Build history of the part. All positions in model axes, mm. A direction names the side the tool comes from. Coordinates: 2 decimals unless noted, no trailing zeros. Loops run counter-clockwise (first coordinate to the right, second up) from the corner with the lowest first, then second, coordinate; pieces in that order, holes last.
Item 1: Drill centre lines: line 1 along Z through (x, y) = (-53.34, -3.75) (3 decimals); line 2 along Z through (x, y) = (-45.72, -4.5) (3 decimals); line 3 along X through (y, z) = (-5.5, -33.5). Where is each one in solid material? Low to high.
Item 2: Cut at A-A (y = -4.5). Count the separate pieces of the cut face and the enclosed holes in it, and give its area (3 significant figures).
Item 3: Flat gauge pins, fed straight in: pin 1 (0.5 mm diameter, centred on y = -2, z = -53.5, fed in from +X); pin 2 (1.5 mm diameter, centred on y = -1, z = 51.5, fed in from +X); pin 3 (3 mm diameter, centred on x = 18, y = -3.5, fed in from +Z) (3 decimals). Where does each tip first touch, or does it go through?
Item 4: Cut at B-B (z = 45.5). List the corners of the cut face in (x, y), and give its area (3 significant figures).
Item 5: Cut at C-C (x = -17). List the corners of the cut face in (y, z) (3 decimals).
Item 6: Mould opens along X. For faces 6 (the face through (-1, -3, 70.485)), 7 (the face through (62, -3, -49.708)), 8 (the face through (63.5, -3, -45)) say: released by +X, released by -X, zero draft, split by the parting line, or undercut.
Item 7: 3-axis set-ups, long thin cutter, end or side, ignore diameter. For faces 1 (the face through (63.5, -3, -63)), 2 (the face through (-62, -3, 52.908)), 3 (the face through (63.5, -3, 45)), 4 (the face through (-56.2, -3.13, -37.19)), 5 (the face through (-63.5, -3, -45)): which of +Z, -Z, +X, -X, +Y, -Y reach the whole face in a straight line?
from build123d import *

# Parameters (mm, degrees)
SKETCH1_R           = 0.4
BOSS_EXTRUDE1_DEPTH = 6.35
SKETCH5_R           = 1.25
CUT_EXTRUDE3_DEPTH  = 6.35
SKETCH4_W           = 3.2
SKETCH4_H           = 6.35
CUT_EXTRUDE4_DEPTH  = 11.43
SKETCH2_W           = 3.2
SKETCH2_H           = 6.35
CUT_EXTRUDE5_DEPTH  = 11.43
FILLET1_R           = 1.27
SKETCH6_W           = 3.81
SKETCH6_H           = 6
CUT_EXTRUDE6_DEPTH  = 6.35
FILLET2_R           = 0.762


with BuildPart() as part:
    # Sketch1 → Boss-Extrude1 (new body)
    with BuildSketch(Plane(origin=(0, 0, 0), x_dir=(1, 0, 0), z_dir=(0, 1, 0))):
        with BuildLine():
            Line((-60.325, -75.565), (-39.37, -75.565))
            ThreePointArc((-39.37, -75.565), (-38.471974388, -75.193025612), (-38.1, -74.295))
            Line((-38.1, -74.295), (-38.1, -71.755))
            ThreePointArc((-38.1, -71.755), (-37.728025612, -70.856974388), (-36.83, -70.485))
            Line((-36.83, -70.485), (36.83, -70.485))
            ThreePointArc((36.83, -70.485), (37.728025612, -70.856974388), (38.1, -71.755))
            Line((38.1, -71.755), (38.1, -74.295))
            ThreePointArc((38.1, -74.295), (38.471974388, -75.193025612), (39.37, -75.565))
            Line((39.37, -75.565), (60.325, -75.565))
            ThreePointArc((60.325, -75.565), (62.57006403, -74.63506403), (63.5, -72.39))
            Line((63.5, -72.39), (63.5, -40.64))
            ThreePointArc((63.5, -40.64), (64.243948776, -38.843948776), (66.04, -38.1))
            Line((66.04, -38.1), (67.31, -38.1))
            ThreePointArc((67.31, -38.1), (69.106051224, -37.356051224), (69.85, -35.56))
            Line((69.85, -35.56), (69.85, 35.56))
            ThreePointArc((69.85, 35.56), (69.106051224, 37.356051224), (67.31, 38.1))
            Line((67.31, 38.1), (66.04, 38.1))
            ThreePointArc((66.04, 38.1), (64.243948776, 38.843948776), (63.5, 40.64))
            Line((63.5, 40.64), (63.5, 72.39))
            ThreePointArc((63.5, 72.39), (62.57006403, 74.63506403), (60.325, 75.565))
            Line((60.325, 75.565), (39.37, 75.565))
            ThreePointArc((39.37, 75.565), (38.471974388, 75.193025612), (38.1, 74.295))
            Line((38.1, 74.295), (38.1, 71.755))
            ThreePointArc((38.1, 71.755), (37.728025612, 70.856974388), (36.83, 70.485))
            Line((36.83, 70.485), (-36.83, 70.485))
            ThreePointArc((-36.83, 70.485), (-37.728025612, 70.856974388), (-38.1, 71.755))
            Line((-38.1, 71.755), (-38.1, 74.295))
            ThreePointArc((-38.1, 74.295), (-38.471974388, 75.193025612), (-39.37, 75.565))
            Line((-39.37, 75.565), (-60.325, 75.565))
            ThreePointArc((-60.325, 75.565), (-62.57006403, 74.63506403), (-63.5, 72.39))
            Line((-63.5, 72.39), (-63.5, 40.64))
            ThreePointArc((-63.5, 40.64), (-64.243948776, 38.843948776), (-66.04, 38.1))
            Line((-66.04, 38.1), (-67.31, 38.1))
            ThreePointArc((-67.31, 38.1), (-69.106051224, 37.356051224), (-69.85, 35.56))
            Line((-69.85, 35.56), (-69.85, -35.56))
            ThreePointArc((-69.85, -35.56), (-69.106051224, -37.356051224), (-67.31, -38.1))
            Line((-67.31, -38.1), (-66.04, -38.1))
            ThreePointArc((-66.04, -38.1), (-64.243948776, -38.843948776), (-63.5, -40.64))
            Line((-63.5, -40.64), (-63.5, -72.39))
            ThreePointArc((-63.5, -72.39), (-62.57006403, -74.63506403), (-60.325, -75.565))
        make_face()
        with Locations(Location((-45.72, 70.485, 0), (0, 0, 270))):
            Circle(SKETCH1_R, mode=Mode.SUBTRACT)
        with Locations(Location((-43.18, 70.485, 0), (0, 0, 270))):
            Circle(SKETCH1_R, mode=Mode.SUBTRACT)
        with Locations(Location((-55.88, 70.485, 0), (0, 0, 270))):
            Circle(SKETCH1_R, mode=Mode.SUBTRACT)
        with Locations(Location((-53.34, 70.485, 0), (0, 0, 270))):
            Circle(SKETCH1_R, mode=Mode.SUBTRACT)
        with BuildLine():
            Line((-53.975, -38.1), (-41.275, -38.1))
            ThreePointArc((-41.275, -38.1), (-39.02993597, -37.17006403), (-38.1, -34.925))
            Line((-38.1, -34.925), (-38.1, 34.925))
            ThreePointArc((-38.1, 34.925), (-39.02993597, 37.17006403), (-41.275, 38.1))
            Line((-41.275, 38.1), (-53.975, 38.1))
            ThreePointArc((-53.975, 38.1), (-56.22006403, 37.17006403), (-57.15, 34.925))
            Line((-57.15, 34.925), (-57.15, -34.925))
            ThreePointArc((-57.15, -34.925), (-56.22006403, -37.17006403), (-53.975, -38.1))
        make_face(mode=Mode.SUBTRACT)
    extrude(amount=-BOSS_EXTRUDE1_DEPTH)

    # Sketch5 → Cut-Extrude3 (cut)
    with BuildSketch(Plane(origin=(0, 0, 0), x_dir=(1, 0, 0), z_dir=(0, 1, 0))):
        with Locations(Location((-11.8, -4.235, 0), (0, 0, 270))):
            Circle(SKETCH5_R)
        with Locations(Location((-11.8, 53.765, 0), (0, 0, 270))):
            Circle(SKETCH5_R)
        with Locations(Location((37.2, -4.235, 0), (0, 0, 270))):
            Circle(SKETCH5_R)
        with Locations(Location((37.2, 53.765, 0), (0, 0, 270))):
            Circle(SKETCH5_R)
    extrude(amount=-CUT_EXTRUDE3_DEPTH, mode=Mode.SUBTRACT)

    # Sketch4 → Cut-Extrude4 (cut)
    with BuildSketch(Plane.ZY.offset(63.5)):
        with Locations((51.308, -3.175)):
            Rectangle(SKETCH4_W, SKETCH4_H)
        with Locations((-51.308, -3.175)):
            Rectangle(SKETCH4_W, SKETCH4_H)
    extrude(amount=-CUT_EXTRUDE4_DEPTH, mode=Mode.SUBTRACT)

    # Sketch2 → Cut-Extrude5 (cut)
    with BuildSketch(Plane(origin=(63.5, 0, 0), x_dir=(0, 0, -1), z_dir=(1, 0, 0))):
        with Locations((51.308, -3.175)):
            Rectangle(SKETCH2_W, SKETCH2_H)
        with Locations((-51.308, -3.175)):
            Rectangle(SKETCH2_W, SKETCH2_H)
    extrude(amount=-CUT_EXTRUDE5_DEPTH, mode=Mode.SUBTRACT)

    # Fillet1
    fillet1_edges = [part.edges().sort_by_distance(p)[0] for p in [
        (-52.07, -3.175, 49.708),
        (-52.07, -3.175, 52.908),
        (-52.07, -3.175, -52.908),
        (-52.07, -3.175, -49.708),
        (52.07, -3.175, -49.708),
        (52.07, -3.175, -52.908),
        (52.07, -3.175, 52.908),
        (52.07, -3.175, 49.708),
    ]]
    fillet(fillet1_edges, radius=FILLET1_R)

    # Sketch6 → Cut-Extrude6 (cut)
    with BuildSketch(Plane(origin=(0, 0, 0), x_dir=(1, 0, 0), z_dir=(0, 1, 0))):
        with Locations((57.785, -51.308)):
            Rectangle(SKETCH6_W, SKETCH6_H)
        with Locations((-57.785, -51.308)):
            Rectangle(SKETCH6_W, SKETCH6_H)
        with Locations((-57.785, 51.308)):
            Rectangle(SKETCH6_W, SKETCH6_H)
        with Locations((57.785, 51.308)):
            Rectangle(SKETCH6_W, SKETCH6_H)
    extrude(amount=-CUT_EXTRUDE6_DEPTH, mode=Mode.SUBTRACT)

    # Fillet2
    fillet2_edges = [part.edges().sort_by_distance(p)[0] for p in [
        (55.88, -3.175, -48.308),
        (59.69, -3.175, -54.308),
        (59.69, -3.175, -48.308),
        (55.88, -3.175, -54.308),
        (-55.88, -3.175, -54.308),
        (-59.69, -3.175, -48.308),
        (-59.69, -3.175, -54.308),
        (-55.88, -3.175, -48.308),
        (-55.88, -3.175, 48.308),
        (-59.69, -3.175, 48.308),
        (-55.88, -3.175, 54.308),
        (-59.69, -3.175, 54.308),
        (55.88, -3.175, 54.308),
        (59.69, -3.175, 48.308),
        (55.88, -3.175, 48.308),
        (59.69, -3.175, 54.308),
    ]]
    fillet(fillet2_edges, radius=FILLET2_R)


solid = part.part
Filled sheet:
1. line 1: z = -75.565 to -70.885, -70.085 to -52.908, -49.708 to -38.1, 38.1 to 49.708, 52.908 to 75.565
1. line 2: z = -75.565 to -70.885, -70.085 to -38.1, 38.1 to 75.565
1. line 3: x = -69.85 to -57.15, -38.1 to 69.85
2. separate pieces: 1
2. enclosed holes: 9
2. area: 17,700 mm2
3. pin 1: stops at x = 63.5
3. pin 2: stops at x = 52.23
3. pin 3: stops at z = 70.485
4. outline: (-63.5, -6.35) - (63.5, -6.35) - (63.5, 0) - (-63.5, 0) - close
4. area: 806 mm2
5. outline: (-6.35, -70.485) - (0, -70.485) - (0, 70.485) - (-6.35, 70.485) - close
6. face 6: undercut
6. face 7: zero draft
6. face 8: released by +X
7. face 1: -Z, +X, +Y, -Y
7. face 2: -X, +Y, -Y
7. face 3: +Z, +X, +Y, -Y
7. face 4: +Y, -Y
7. face 5: -Z, -X, +Y, -Y
